Verification items for the finished model (mm, model axes). Coordinates: 2 decimals unless noted, no trailing zeros. Order: outer loops, then holes, each group sorted by start corner. A loop starts at its lowest first (then second) coordinate and runs counter-clockwise, first axis right, second up.
Q1. Depth check by flat-ended pin: P1, Ø3, axis at x = 116, z = 6.5, coming from the -Y side; P2, Ø1.9, axis at y = -2.5, z = 6, coming from the +X side; P3, Ø4, axis at y = -3, z = 6.5, coming from the -X side. Enter the tip coordinate at first touch or a pass-through.
Q2. Cross-section at A-A, the plane z = 6. Record the boundary of the cut face in (x, y).
Q3. Cross-section at C-C, the plane y = 0.5. Count the separate pieces of the cut face and the enclosed holes in it, and give its area (3 significant figures).
Q4. Thickness scan on line 1 (X direction, y = 2, z = 1); line 2 (X direction, y = 8, z = 6.75); line 3 (X direction, y = -2.5, z = 0.5). Record the ranges inside material, lowest first.
Q5. Cross-section at B-B, the plane x = -41. Record the boundary of the cut face in (y, z).
from build123d import *

# Parameters (mm, degrees)
F0_W     = 6.35
F0_H     = 19.05
F0_R     = 17.5576306553
F1_DEPTH = 3.81
F2_R     = 1.27
F3_W     = 7.62
F3_H     = 19.304
F4_DEPTH = 5.08
F5_R     = 1.27


# Not quite as in the source:
# - a feature names something its author has since deleted; it is built from what else it names


with BuildPart() as f1:
    # F0 (on Top) → F1 (new body)
    with BuildSketch(Plane.XY):
        with BuildLine():
            ThreePointArc((127, 11.43), (125.1401280605, 15.9201280605), (120.65, 17.78))
            Line((120.65, 17.78), (-120.65, 17.78))
            ThreePointArc((-120.65, 17.78), (-125.1401280605, 15.9201280605), (-127, 11.43))
            Line((-127, 11.43), (-127, -11.43))
            ThreePointArc((-127, -11.43), (-125.1401280605, -15.9201280605), (-120.65, -17.78))
            Line((-120.65, -17.78), (120.65, -17.78))
            ThreePointArc((120.65, -17.78), (125.1401280605, -15.9201280605), (127, -11.43))
            Line((127, -11.43), (127, 11.43))
        make_face()
        with Locations((-117.475, 0)):
            Rectangle(F0_W, F0_H, mode=Mode.SUBTRACT)
        with Locations((-104.775, 0)):
            Rectangle(F0_W, F0_H, mode=Mode.SUBTRACT)
        with Locations((-92.075, 0)):
            Rectangle(F0_W, F0_H, mode=Mode.SUBTRACT)
        with Locations((-79.375, 0)):
            Rectangle(F0_W, F0_H, mode=Mode.SUBTRACT)
        with Locations((-66.675, 0)):
            Rectangle(F0_W, F0_H, mode=Mode.SUBTRACT)
        with Locations((4.1378471069, 0)):
            Circle(F0_R, mode=Mode.SUBTRACT)
        with Locations((4.1378471069, 0)):
            Circle(F0_R)
    extrude(amount=F1_DEPTH)

    # F2
    f2_edges = [f1.edges().sort_by_distance(p)[0] for p in [
        (0, -17.78, 0),
        (0, -17.78, 3.81),
    ]]
    fillet(f2_edges, radius=F2_R)

    # F3 (on face) → F4 (join)
    with BuildSketch(Plane.XY.offset(3.81)):
        with Locations((102.87, 0)):
            Rectangle(F3_W, F3_H)
        with Locations((115.57, 0)):
            Rectangle(F3_W, F3_H)
    extrude(amount=F4_DEPTH)

    # F5
    f5_edges = [f1.edges().sort_by_distance(p)[0] for p in [
        (106.68, 0, 8.89),
        (102.87, -9.652, 8.89),
        (99.06, 0, 8.89),
        (102.87, 9.652, 8.89),
        (111.76, 0, 8.89),
        (119.38, 0, 8.89),
        (115.57, -9.652, 8.89),
        (115.57, 9.652, 8.89),
        (119.38, -9.652, 6.35),
        (111.76, -9.652, 6.35),
        (106.68, -9.652, 6.35),
        (99.06, -9.652, 6.35),
        (106.68, 9.652, 6.35),
        (119.38, 9.652, 6.35),
        (111.76, 9.652, 6.35),
        (99.06, 9.652, 6.35),
    ]]
    fillet(f5_edges, radius=F5_R)


solid = f1.part
Check values:
1. P1: stops at y = -9.65
1. P2: stops at x = 119.38
1. P3: stops at x = 99.06
2. outline: (99.06, -8.38) arc R1.27 ccw to (100.33, -9.65) - (105.41, -9.65) arc R1.27 ccw to (106.68, -8.38) - (106.68, 8.38) arc R1.27 ccw to (105.41, 9.65) - (100.33, 9.65) arc R1.27 ccw to (99.06, 8.38) - close; (111.76, -8.38) arc R1.27 ccw to (113.03, -9.65) - (118.11, -9.65) arc R1.27 ccw to (119.38, -8.38) - (119.38, 8.38) arc R1.27 ccw to (118.11, 9.65) - (113.03, 9.65) arc R1.27 ccw to (111.76, 8.38) - close
3. separate pieces: 6
3. enclosed holes: 0
3. area: 921 mm2
4. line 1: x = -126.97 to -120.65, -114.3 to -107.95, -101.6 to -95.25, -88.9 to -82.55, -76.2 to -69.85, -63.5 to 126.97
4. line 2: x = 99.06 to 106.68, 111.76 to 119.38
4. line 3: x = -126.74 to -120.65, -114.3 to -107.95, -101.6 to -95.25, -88.9 to -82.55, -76.2 to -69.85, -63.5 to 126.74
5. outline: (-17.78, 1.27) arc R1.27 ccw to (-16.51, 0) - (16.51, 0) arc R1.27 ccw to (17.78, 1.27) - (17.78, 2.54) arc R1.27 ccw to (16.51, 3.81) - (-16.51, 3.81) arc R1.27 ccw to (-17.78, 2.54) - close
